Geometry check sheet. Reference: the model listing, model coordinates, mm. A direction names the side the tool comes from. Round coordinates to 2 decimals unless told otherwise and drop trailing zeros. Write each loop counter-clockwise with the first axis right and the second up, starting at its lowest first coordinate (ties: lowest second). Pieces come first, ordered by that corner, then holes. Notation, with made-up numbers: (-28, -22) -> (-16, -22) arc R16 ccw to (-16, -16) -> close; hole circle Ø5 at (75.5, 61.25). An arc over 180 degrees is marked (long way). Return JSON: item names as keys, results as strings. Group by question number.
Autodesk Inventor part; units mm, degrees
ref_plane "rod_cp_XY" through (0, 0, 0) normal (1, 0, 0) x (0, 0, -1)
ref_plane "rod_cp_YZ" through (0, 0, 0) normal (0, 0, -1) x (0, 1, 0)
ref_plane "rod_cp_ZX" through (0, 0, 0) normal (0, 1, 0) x (1, 0, 0)
sketch "Sketch_1" plane through (0, 0, 0) normal (0, 0, 1) x (1, 0, 0)
  line L0 (112.7252, 0) -> (0, 0)
  line L1 (0, 0) -> (0, 3.175)
  line L2 (0, 3.175) -> (91.2876, 3.175)
  line L3 (91.2876, 3.175) -> (91.2876, 9.6203)
  line L4 (91.2876, 9.6203) -> (112.7252, 9.6203)
  line L5 (112.7252, 9.6203) -> (112.7252, 0)
  line L6 (112.7252, 0) -> (0, 0)
revolve "Revolution1" add sketch "Sketch_1" angle 360 about axis through (112.7252, 0, 0) along (1, 0, 0)
sketch "Sketch_3" plane through (0, 0, 0) normal (0, 0, 1) x (1, 0, 0)
  line L0 (0, 0) -> (-12.7, 0)
  line L1 (-12.7, 0) -> (-12.7, 2.634)
  line L2 (-12.7, 2.634) -> (-12.159, 3.175)
  line L3 (-12.159, 3.175) -> (0, 3.175)
  line L4 (0, 3.175) -> (0, 0)
  line L5 (0, 0) -> (-12.7, 0)
revolve "Revolution2" add sketch "Sketch_3" angle 360 about axis through (0, 0, 0) along (1, 0, 0)
thread "Thread1"
sketch "Sketch_30" plane through (0, 0, 0) normal (0, 0, 1) x (1, 0, 0)
  line L0 (0, 0) -> (-0.254, 0)
  line L1 (-0.254, 3.429) -> (-0.254, 2.921)
  line L2 (-0.254, 2.921) -> (0, 2.921)
  line L3 (0, 2.921) -> (0, 3.429)
  line L4 (0, 3.429) -> (-0.254, 3.429)
revolve "Revolution3" cut sketch "Sketch_30" angle 360 about axis through (0, 0, 0) along (1, 0, 0)
ref_plane "rod_cp_XY" through (0, 0, 0) normal (1, 0, 0) x (0, 0, -1)
ref_plane "rod_cp_YZ" through (0, 0, 0) normal (0, 0, -1) x (0, 1, 0)
ref_plane "rod_cp_ZX" through (0, 0, 0) normal (0, 1, 0) x (1, 0, 0)
ref_plane "to_rod_clevis_XY" through (-12.7, 0, 0) normal (1, 0, 0) x (0, 0, -1)
ref_plane "to_rod_clevis_YZ" through (-12.7, 0, 0) normal (0, 0, -1) x (0, 1, 0)
ref_plane "to_rod_clevis_ZX" through (-12.7, 0, 0) normal (0, 1, 0) x (1, 0, 0)
ref_plane "rl2_XY" through (0, 0, 0) normal (1, 0, 0) x (0, 0, -1)
ref_plane "rl2_YZ" through (0, 0, 0) normal (0, 0, -1) x (0, 1, 0)
ref_plane "rl2_ZX" through (0, 0, 0) normal (0, 1, 0) x (1, 0, 0)
ref_plane "rl1_XY" through (-12.7, 0, 0) normal (1, 0, 0) x (0, 0, -1)
ref_plane "rl1_YZ" through (-12.7, 0, 0) normal (0, 0, -1) x (0, 1, 0)
ref_plane "rl1_ZX" through (-12.7, 0, 0) normal (0, 1, 0) x (1, 0, 0)
ref_plane "thd1_XY" through (-12.7, 3.175, 0) normal (1, 0, 0) x (0, 0, -1)
ref_plane "thd1_YZ" through (-12.7, 3.175, 0) normal (0, 0, -1) x (0, 1, 0)
ref_plane "thd1_ZX" through (-12.7, 3.175, 0) normal (0, 1, 0) x (1, 0, 0)
ref_plane "thd2_XY" through (-12.7, -3.175, 0) normal (1, 0, 0) x (0, 0, -1)
ref_plane "thd2_YZ" through (-12.7, -3.175, 0) normal (0, 0, -1) x (0, 1, 0)
ref_plane "thd2_ZX" through (-12.7, -3.175, 0) normal (0, 1, 0) x (1, 0, 0)
ref_plane "dia1_XY" through (0, 3.175, 0) normal (1, 0, 0) x (0, 0, -1)
ref_plane "dia1_YZ" through (0, 3.175, 0) normal (0, 0, -1) x (0, 1, 0)
ref_plane "dia1_ZX" through (0, 3.175, 0) normal (0, 1, 0) x (1, 0, 0)
ref_plane "dia2_XY" through (0, -3.175, 0) normal (1, 0, 0) x (0, 0, -1)
ref_plane "dia2_YZ" through (0, -3.175, 0) normal (0, 0, -1) x (0, 1, 0)
ref_plane "dia2_ZX" through (0, -3.175, 0) normal (0, 1, 0) x (1, 0, 0)
ref_plane "hh1_XY" through (142.8496, 0, 0) normal (0, 0, 1) x (1, 0, 0)
ref_plane "hh1_YZ" through (142.8496, 0, 0) normal (1, 0, 0) x (0, 1, 0)
ref_plane "hh1_ZX" through (142.8496, 0, 0) normal (0, 1, 0) x (0, 0, 1)
ref_plane "hh2_XY" through (149.2504, 0, 0) normal (0, 0, 1) x (1, 0, 0)
ref_plane "hh2_YZ" through (149.2504, 0, 0) normal (1, 0, 0) x (0, 1, 0)
ref_plane "hh2_ZX" through (149.2504, 0, 0) normal (0, 1, 0) x (0, 0, 1)
ref_plane "dia12_XY" through (0, 0, 10.9537) normal (1, 0, 0) x (0, 0, -1)
ref_plane "dia12_YZ" through (0, 0, 10.9537) normal (0, 0, -1) x (0, 1, 0)
ref_plane "dia12_ZX" through (0, 0, 10.9537) normal (0, 1, 0) x (1, 0, 0)
ref_plane "dia22_XY" through (0, 0, -10.9537) normal (1, 0, 0) x (0, 0, -1)
ref_plane "dia22_YZ" through (0, 0, -10.9537) normal (0, 0, -1) x (0, 1, 0)
ref_plane "dia22_ZX" through (0, 0, -10.9537) normal (0, 1, 0) x (1, 0, 0)
properties part number "042-DXP0_rod"
1) Sectioned sample at A-A on z = 0. Enter the section's corners in (x, y) (3 decimals).
2) Sectioned sample at D-D on z = -5.75. Enter the section's corners in (x, y), and give its area (3 significant figures).
3) Tool access check on faces 1 (the face through (112.725, 0, 0)), 2 (the face through (-6.12, -0.69, -3.1)). Record the directions out of +Z, -Z, +X, -X, +Y, -Y that give a thin tool (end or side, any length) a straight path to the whole face; none if there is none.
4) Material ranges on probe 1 along X at (y, z) = (3, 7.25); probe 2 along Y at (x, z) = (106, 2.5); probe 3 along Y at (x, z) = (82, 0.75), recorded low to high. Write a range as [from, to].
5) Go/stop test with flat-tipped pins: P1, Ø5, axis at x = 82.5, z = -3, coming from the -Y side; P2, Ø1, axis at x = 43, z = 4, coming from the -Y side; P3, Ø5, axis at x = 24.5, z = -5, coming from the -Y side; P4, Ø8, axis at x = 23.5, y = -3.5, coming from the +Z side (3 decimals). Record where each tip stops, or that it passes through.
6) Sectioned sample at C-C on x = 34. Enter the section's corners in (y, z) (3 decimals).
Evaluation:
{
 "1": {"outline": "(-12.7, -2.634) -> (-12.159, -3.175) -> (-0.254, -3.175) -> (-0.254, -2.921) -> (0, -2.921) -> (0, -3.175) -> (91.288, -3.175) -> (91.288, -9.62) -> (112.725, -9.62) -> (112.725, 9.62) -> (91.288, 9.62) -> (91.288, 3.175) -> (0, 3.175) -> (0, 2.921) -> (-0.254, 2.921) -> (-0.254, 3.175) -> (-12.159, 3.175) -> (-12.7, 2.634) -> close"},
 "2": {"outline": "(91.29, -7.71) -> (112.73, -7.71) -> (112.73, 7.71) -> (91.29, 7.71) -> close", "area": "331 mm2"},
 "3": {"face 1": "+Z, -Z, +X, +Y, -Y", "face 2": "-X"},
 "4": {"probe 1": "x = [91.29, 112.73]", "probe 2": "y = [-9.29, 9.29]", "probe 3": "y = [-3.09, 3.09]"},
 "5": {"P1": "stops at y = -3.14", "P2": "passes through", "P3": "stops at y = -1.96", "P4": "stops at z = 3.175"},
 "6": {"outline": "circle Ø6.35 at (0, 0)"}
}
